Work out the finished part from the listing and answer in its coordinate system (mm). Give positions to 0.01 mm unless a question says otherwise; leave off trailing zeros. Loops run counter-clockwise (first coordinate to the right, second up) from the corner with the lowest first, then second, coordinate; pieces in that order, holes last. Notation, with made-up numbers: (56.25, 88) -> (60.25, 88) arc R21 cw to (60.25, 123) -> close; hole circle Ø9 at (28, 69). An arc over 180 degrees is marked (long way). Answer as CSV lines item,"result". Start each with the question number.
1. A flat-ended cylindrical pin translates along its axis: pin 1 Ø1 at (x, z) = (-3.5, -0.5) entering from +Y. Find the tip coordinate at first contact, or state that the pin passes through.
2. Find the intervals of material crossed by line 1 along Y through (x, z) = (0, -0.75); line 2 along X through (y, z) = (2.5, -0.6); line 3 along X through (y, z) = (-1, 0.2), in increasing order.
3. Find section A-A, the plane x = 0. Give the vertices of the cut face in (y, z).
4. Determine the mould class of faces 1 (the face through (-3, 0, 0)), 2 (the face through (-2.4, 2.3, 2)), 3 (the face through (-2.666, 4.653, -1.867)) for opening direction Y: +Y half, -Y half, draft (parallel to the pull), parting line (faces both ways), or undercut.
5. Find section C-C, the plane y = 2. Give the vertices of the cut face in (x, z).
6. Find section B-B, the plane z = -0.55. Give the vertices of the cut face in (x, y), and give its area (3 significant figures).
from build123d import *

# Parameters (mm, degrees)
SKETCH_R  = 3
PAD_DEPTH = 2


with BuildPart() as part:
    # Sketch → Pad (new body, symmetric)
    with BuildSketch(Plane.XY):
        Polygon((2.886751, 5), (-2.886751, 5), (-5.773503, 0), (-2.886751, -5), (2.886751, -5), (5.773503, 0), align=None)
        Circle(SKETCH_R, mode=Mode.SUBTRACT)
    extrude(amount=PAD_DEPTH, both=True)

    # Sketch001 → Groove (revolve, cut)
    with BuildSketch(Plane.XZ):
        Polygon((4.606088, 2.527526), (6.100964, 1.220869), (6.100964, -1.220869), (4.606088, -2.527526), (7.425626, -2.527526), (7.425626, 2.527526), align=None)
    revolve(axis=Axis((0, 0, 0), (0, 0, 1)), mode=Mode.SUBTRACT)


solid = part.part
Resolved:
1,pin 1,"stops at y = 4.8"
2,line 1,"y = -5 to -3, 3 to 5"
2,line 2,"x = -4.33 to -1.66, 1.66 to 4.33"
2,line 3,"x = -5.2 to -2.83, 2.83 to 5.2"
3,outline,"(-5, -2) -> (-3, -2) -> (-3, 2) -> (-5, 2) -> close; (3, -2) -> (5, -2) -> (5, 2) -> (3, 2) -> close"
4,face 1,"undercut"
4,face 2,"draft"
4,face 3,"+Y half"
5,outline,"(-4.62, -2) -> (-2.24, -2) -> (-2.24, 2) -> (-4.62, 2) -> close; (2.24, -2) -> (4.62, -2) -> (4.62, 2) -> (2.24, 2) -> close"
6,outline,"(-5.77, 0) -> (-2.89, -5) -> (2.89, -5) -> (5.77, 0) -> (2.89, 5) -> (-2.89, 5) -> close; hole circle Ø6 at (0, 0)"
6,area,"58.3 mm^2"
